```python
from build123d import *

# Parameters (mm, degrees)
F1_DEPTH      = 6.35
F1_DEPTH_BACK = 6.35
F2_R          = 1.90452
F3_DEPTH      = 15.357033
F4_DEPTH      = 14.148086
F5_R          = 5.708941
F6_DEPTH      = 15.330171


with BuildPart() as f1:
    # F0 (on Front) → F1 (new body, two sides)
    with BuildSketch(Plane.XZ) as f1_sk:
        with BuildLine():
            Line((10.257333, -4.399853), (18.612302, -4.399853))
            Line((18.612302, -4.399853), (18.612302, 4.399853))
            Line((18.612302, 4.399853), (-18.612302, 4.399853))
            Line((-18.612302, 4.399853), (-18.612302, -4.399853))
            Line((-18.612302, -4.399853), (-10.257333, -4.399853))
            ThreePointArc((-10.257333, -4.399853), (0, -14.657186), (10.257333, -4.399853))
        make_face()
    extrude(amount=F1_DEPTH)
    extrude(f1_sk.sketch, amount=-F1_DEPTH_BACK)

    # F2 (on face) → F3 (cut)
    with BuildSketch(Plane.XZ.offset(6.35)):
        with Locations((-15.430572, 0)):
            Circle(F2_R)
    extrude(amount=-F3_DEPTH, mode=Mode.SUBTRACT)

    # F2 (on face) → F4 (cut)
    with BuildSketch(Plane.XZ.offset(6.35)):
        with Locations((15.430572, 0)):
            Circle(F2_R)
    extrude(amount=-F4_DEPTH, mode=Mode.SUBTRACT)

    # F5 (on face) → F6 (cut)
    with BuildSketch(Plane.XZ.offset(6.35)):
        with Locations((0, -7.068473)):
            Circle(F5_R)
    extrude(amount=-F6_DEPTH, mode=Mode.SUBTRACT)


solid = f1.part
```
Geometry: final body of the model. Coordinates: model frame, mm. A direction names the side the tool comes from. Round coordinates to 2 decimals unless told otherwise and drop trailing zeros. Write each loop counter-clockwise with the first axis right and the second up, starting at its lowest first coordinate (ties: lowest second). Pieces come first, ordered by that corner, then holes.
Item 1: Section query B-B (z = -7.75). Return loops of the section in (x, y).
Item 2: Pin query (flat end, axial travel): P1, Ø6.5, axis at x = 16.5, y = 1.5, coming from the -Z side. Return the tip coordinate at first contact, or that it passes through.
Item 3: Material intervals for L1, parallel to Z at x = 0, y = 3; L2, parallel to X at y = 2.75, z = 0.75; L3, parallel to Z at x = 15.5, y = 1.5, sorted ascending.
Item 4: Section query A-A (x = 0). Return loops of the section in (y, z), plus the area to 3 significant figures.
Item 5: Section query C-C (z = 0). Return loops of the section in (x, y), plus the area to 3 significant figures.
Item 6: Set-up query: faces 4 (the face through (-14, 0, -4.4)), 5 (the face through (0, 6.35, -1)), 6 (the face through (14, 0, -4.4)). Return all of +Z, -Z, +X, -X, +Y, -Y with unobstructed straight access to the full face (end or side cutting, diameter ignored); none if empty.
Item 7: Section query D-D (y = 2.75). Return loops of the section in (x, z), plus the area to 3 significant figures.
Item 8: Mould query, pull axis Z, two halves, no side actions, for faces 1 (the face through (-13.67, -0.09, -0.73)), 2 (the face through (0, 0, 4.4)), 3 (the face through (18.612, 0, 0)). Classes: +Z half, -Z half, draft (parallel to the pull), parting line (faces both ways), or undercut.
Completed:
1. outline: (-9.69, -6.35) - (-5.67, -6.35) - (-5.67, 6.35) - (-9.69, 6.35) - close; (5.67, -6.35) - (9.69, -6.35) - (9.69, 6.35) - (5.67, 6.35) - close
2. P1: stops at z = -4.4
3. L1: z = -14.66 to -12.78, -1.36 to 4.4
3. L2: x = -18.61 to -17.18, -13.68 to 13.68, 17.18 to 18.61
3. L3: z = -4.4 to -1.9, 1.9 to 4.4
4. outline: (-6.35, -14.66) - (6.35, -14.66) - (6.35, -12.78) - (-6.35, -12.78) - close; (-6.35, -1.36) - (6.35, -1.36) - (6.35, 4.4) - (-6.35, 4.4) - close
4. area: 97.0 mm2
5. outline: (-18.61, -6.35) - (-17.34, -6.35) - (-17.34, 6.35) - (-18.61, 6.35) - close; (-13.53, -6.35) - (13.53, -6.35) - (13.53, 6.35) - (-13.53, 6.35) - close; (17.34, -6.35) - (18.61, -6.35) - (18.61, 6.35) - (17.34, 6.35) - close
5. area: 376 mm2
6. face 4: -Z, -X, +Y, -Y
6. face 5: +Z, -Z, +X, -X, +Y
6. face 6: -Z, +X, +Y, -Y
7. outline: (-18.61, -4.4) - (-10.26, -4.4) arc R10.26 ccw to (10.26, -4.4) - (18.61, -4.4) - (18.61, 4.4) - (-18.61, 4.4) - close; hole circle Ø3.81 at (-15.43, 0); hole circle Ø11.42 at (0, -7.07); hole circle Ø3.81 at (15.43, 0)
7. area: 368 mm2
8. face 1: undercut
8. face 2: +Z half
8. face 3: draft
